Could you check a few things on this model? Use its own coordinates, in mm. Face numbers are marked on the shaded views. A direction names the side the tool comes from. Coordinates: 2 decimals unless noted, no trailing zeros. Loops run counter-clockwise (first coordinate to the right, second up) from the corner with the lowest first, then second, coordinate; pieces in that order, holes last. Notation, with made-up numbers: (37.5, 75.25) - (45.5, 75.25) arc R14 ccw to (45.5, 91.25) - close; hole circle Ø1 at (88.5, 65.25). An arc over 180 degrees is marked (long way). Put each result on its own line as item: value. Start each with the question number.
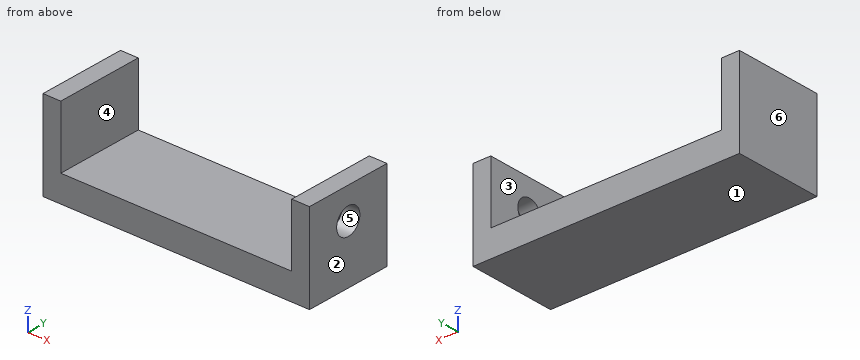
```python
from build123d import *

# Parameters (mm, degrees)
SKETCH_1_W          = 30
SKETCH_1_H          = 10
EXTRUDE_1_DEPTH     = 1.5
SKETCH_2_W          = 2
SKETCH_2_H          = 10
EXTRUDE_2_DEPTH     = 7
CUT_EXTRUDE_1_REACH = 33.579
SKETCH_3_R          = 1.5


with BuildPart() as part:
    # 草图1 → 凸台-拉伸1 (new, symmetric)
    with BuildSketch(Plane.XY):
        Rectangle(SKETCH_1_W, SKETCH_1_H)
    extrude(amount=EXTRUDE_1_DEPTH, both=True)

    # 草图2 → 凸台-拉伸2 (add)
    with BuildSketch(Plane.XY.offset(1.5)):
        with Locations((-14, 0)):
            Rectangle(SKETCH_2_W, SKETCH_2_H)
        with Locations((14, 0)):
            Rectangle(SKETCH_2_W, SKETCH_2_H)
    extrude(amount=EXTRUDE_2_DEPTH)

    # 草图3 → 切除-拉伸1 (cut, up to next)
    with BuildSketch(Plane(origin=(15, 0, 0), x_dir=(0, 0, -1), z_dir=(1, 0, 0)), mode=Mode.PRIVATE) as cut_extrude_1_sk1:
        with Locations((-5, 0)):
            Circle(SKETCH_3_R)
    cut_extrude_1_tool1 = extrude(cut_extrude_1_sk1.sketch, amount=-CUT_EXTRUDE_1_REACH, mode=Mode.PRIVATE) & part.part
    add(cut_extrude_1_tool1.solids().sort_by_distance((15, 0, 5))[0], mode=Mode.SUBTRACT)


solid = part.part
```
(1) I want a section at B-B on z = 5. List the corners of the cut face in (x, y) for me, and give its area (3 significant figures).
(2) Which directions (+Z, -Z, +X, -X, +Y, -Y) give clear straight access to the entire face, cutting with the end or side of a thin tool? Please do the marked faces 4, 5 and 6.
(3) If we mould it in two halves opening along X, with no side actions, what happens to the marked faces 1, 2 and 3? For each: pulls with the +X half, pulls with the -X half, needs draft (parallel to the pull), parting line crosses it, or undercut.
(4) For pin 1 Ø4 at (y, z) = (0, 5) entering from +X, with a flat end and sliding along its axis, tell me the tip position at first contact or that it passes through.
(5) I want a section at A-A on y = 0. List the corners of the cut face in (x, z) for me.
(6) I want a section at D-D on x = -3. List the corners of the cut face in (y, z) for me.
(7) I need wall thicknesses on L1, parallel to X at y = -4, z = 3; L2, parallel to Y at x = 13.4, z = 5; L3, parallel to Z at x = -11.5, y = -1.75. Which ranges of each line are inside material? Lowest first, please. Write a range as [from, to].
(8) I want a section at C-C on y = -3.75. List the corners of the cut face in (x, z) for me, and give its area (3 significant figures).
Answer sheet:
1. outline: (-15, -5) - (-13, -5) - (-13, 5) - (-15, 5) - close; (13, -5) - (15, -5) - (15, -1.5) - (13, -1.5) - close; (13, 1.5) - (15, 1.5) - (15, 5) - (13, 5) - close
1. area: 34.0 mm^2
2. face 4: +Z, +Y, -Y
2. face 5: +X
2. face 6: +Z, -Z, -X, +Y, -Y
3. face 1: needs draft
3. face 2: pulls with the +X half
3. face 3: undercut
4. pin 1: stops at x = 15
5. outline: (-15, -1.5) - (15, -1.5) - (15, 3.5) - (13, 3.5) - (13, 1.5) - (-13, 1.5) - (-13, 8.5) - (-15, 8.5) - close; (13, 6.5) - (15, 6.5) - (15, 8.5) - (13, 8.5) - close
6. outline: (-5, -1.5) - (5, -1.5) - (5, 1.5) - (-5, 1.5) - close
7. L1: x = [-15, -13], [13, 15]
7. L2: y = [-5, -1.5], [1.5, 5]
7. L3: z = [-1.5, 1.5]
8. outline: (-15, -1.5) - (15, -1.5) - (15, 8.5) - (13, 8.5) - (13, 1.5) - (-13, 1.5) - (-13, 8.5) - (-15, 8.5) - close
8. area: 118 mm^2
